Work out the finished part from the listing and answer in its coordinate system (mm). A direction names the side the tool comes from. Coordinates: 2 decimals unless noted, no trailing zeros. Write item = value, one per line. Start each with the question number.
Q1. Determine the mould class of faces 1 (the flat face through (17.5, -1, 48)), 2 (the cylindrical face through (0.245, 37.269, 35.107)), 3 (the cylindrical face through (0.245, 42.898, -55.946)) for opening direction Y: released by +Y, released by -Y, zero draft, split by the parting line, or undercut.
Q2. Find section A-A on x = -3. Give the number of separate pieces and of enclosed holes in the cut face, and give its area (3 significant figures).
Q3. Each of these flat-tipped pins is pushed along its axis until it touches: P1, Ø12, axis at x = -13.5, z = 45.5, coming from the -Y side; P2, Ø3, axis at x = -10, y = -50.5, coming from the +Z side; P3, Ø4, axis at x = 7.5, z = 46, coming from the +Y side. Where does it stop, or does it pass through?
Q4. Straight lines are drawn through the part: line 1 along Z through (x, y) = (15, -31); line 2 along Y through (x, z) = (8, -28); line 3 along Y through (x, z) = (-2, -62). For each, find the intervals that lie inside material, in ascending order.
Q5. A tool of negligible diameter and unlimited length cuts with its end or side. For faces 4 (the cylindrical face through (-11.239, 19.653, -45.292)), 5 (the cylindrical face through (11.2, 10.1, 55.6)), 6 (the cylindrical face through (0.245, 52.184, 26.527)), from which of +Z, -Z, +X, -X, +Y, -Y can it reach the whole face along a straight path? Write none if from no direction.
```python
from build123d import *

# Parameters (mm, degrees)
SKETCH1_W             = 35
SKETCH1_H             = 5
SKETCH7_R             = 46.2
REINFORCEMENT_DEPTH   = 35
SKETCH8_R             = 4
INSERTS_HOLES_A_DEPTH = 12.7


with BuildPart() as part:
    # Sketch1 → Body (revolve)
    with BuildSketch(Plane(origin=(0, 0, 0), x_dir=(1, 0, 0), z_dir=(0, 1, 0)), mode=Mode.PRIVATE) as body_sk:
        with Locations((0, 68)):
            Rectangle(SKETCH1_W, SKETCH1_H)
    revolve(body_sk.sketch.rotate(Axis((-1000, 0, 0), (1, 0, 0)), 180), axis=Axis((-1000, 0, 0), (1, 0, 0)))

    # Sketch7 → Reinforcement (add)
    with BuildSketch(Plane.ZY.offset(-17.5)):
        with BuildLine():
            ThreePointArc((15.227788826, 63.705293716), (7.666591863, 65.049776089), (0, 65.5))
            ThreePointArc((0, 65.5), (3.008755476, 58.35), (0, 51.2))
            ThreePointArc((0, 51.2), (-4.264821355, 51.022066783), (-8.5, 50.48950386))
            ThreePointArc((-8.5, 50.48950386), (-7.314547286, 58.179485578), (-12, 64.391381411))
            ThreePointArc((-12, 64.391381411), (-19.454347387, 62.544211305), (-26.641250121, 59.837227476))
            ThreePointArc((-26.641250121, 59.837227476), (-20.984448226, 54.529148555), (-20.824916125, 46.773527431))
            ThreePointArc((-20.824916125, 46.773527431), (-24.648652343, 44.876318228), (-28.3010677, 42.667195444))
            ThreePointArc((-28.3010677, 42.667195444), (-30.345900107, 50.17451037), (-37.15287981, 53.943614282))
            ThreePointArc((-37.15287981, 53.943614282), (-43.211453237, 49.22418419), (-48.675986069, 43.828054717))
            ThreePointArc((-48.675986069, 43.828054717), (-41.349250191, 41.279711944), (-38.049015064, 34.259487046))
            ThreePointArc((-38.049015064, 34.259487046), (-40.770507414, 30.971046563), (-43.208623688, 27.467341316))
            ThreePointArc((-43.208623688, 27.467341316), (-48.130171117, 33.493906497), (-55.881689177, 34.168506182))
            ThreePointArc((-55.881689177, 34.168506182), (-59.496906258, 27.392848441), (-62.294201817, 20.240613132))
            ThreePointArc((-62.294201817, 20.240613132), (-54.564391152, 20.892638123), (-48.694093634, 15.821670112))
            ThreePointArc((-48.694093634, 15.821670112), (-49.842771366, 11.710599583), (-50.645016102, 7.518134342))
            ThreePointArc((-50.645016102, 7.518134342), (-57.592298291, 11.021901908), (-64.948046817, 8.485352952))
            ThreePointArc((-64.948046817, 8.485352952), (-65.494803675, 0.82504034), (-65.141184147, -6.846614344))
            ThreePointArc((-65.141184147, -6.846614344), (-58.344853181, -3.106962633), (-50.919521043, -5.351857319))
            ThreePointArc((-50.919521043, -5.351857319), (-50.29676734, -9.574716451), (-49.324425137, -13.73102636))
            ThreePointArc((-49.324425137, -13.73102636), (-57.096193882, -13.355889651), (-62.784297127, -18.664994891))
            ThreePointArc((-62.784297127, -18.664994891), (-60.168054535, -25.88542473), (-56.724663948, -32.75))
            ThreePointArc((-56.724663948, -32.75), (-52.036960049, -26.569341324), (-44.340500674, -25.6))
            ThreePointArc((-44.340500674, -25.6), (-42.05399531, -29.204477028), (-39.475192967, -32.605967862))
            ThreePointArc((-39.475192967, -32.605967862), (-46.727638847, -35.424326556), (-49.764572087, -42.587995551))
            ThreePointArc((-49.764572087, -42.587995551), (-44.437702156, -48.120064704), (-38.499934025, -52.990613132))
            ThreePointArc((-38.499934025, -52.990613132), (-36.731403783, -45.437639525), (-30.094604917, -41.421670112))
            ThreePointArc((-30.094604917, -41.421670112), (-26.539705442, -43.784518212), (-22.800341312, -45.843041305))
            ThreePointArc((-22.800341312, -45.843041305), (-28.279450549, -51.367575579), (-28.140100436, -59.14714488))
            ThreePointArc((-28.140100436, -59.14714488), (-21.023667371, -62.034308332), (-13.618215749, -64.068667848))
            ThreePointArc((-13.618215749, -64.068667848), (-15.074654109, -56.449357065), (-10.64507857, -50.081157158))
            ThreePointArc((-10.64507857, -50.081157158), (-6.436459398, -50.793818427), (-2.18310351, -51.153436435))
            ThreePointArc((-2.18310351, -51.153436435), (-4.94148834, -58.428904124), (-1.649949774, -65.479215525))
            ThreePointArc((-1.649949774, -65.479215525), (6.025550497, -65.222256487), (13.618215749, -64.068667848))
            ThreePointArc((13.618215749, -64.068667848), (9.18864021, -57.700467941), (10.64507857, -50.081157158))
            ThreePointArc((10.64507857, -50.081157158), (14.77970895, -49.020405989), (18.811612722, -47.618937691))
            ThreePointArc((18.811612722, -47.618937691), (19.250902095, -55.387344337), (25.125492192, -60.489334945))
            ThreePointArc((25.125492192, -60.489334945), (32.032895944, -57.132683969), (38.499934025, -52.990613132))
            ThreePointArc((38.499934025, -52.990613132), (31.86313516, -48.974643718), (30.094604917, -41.421670112))
            ThreePointArc((30.094604917, -41.421670112), (33.440331351, -38.770920019), (36.553630216, -35.850692016))
            ThreePointArc((36.553630216, -35.850692016), (40.114636669, -42.768809535), (47.556508301, -45.040298825))
            ThreePointArc((47.556508301, -45.040298825), (52.501462672, -39.164351358), (56.724663948, -32.75))
            ThreePointArc((56.724663948, -32.75), (49.028204573, -31.780658676), (44.340500674, -25.6))
            ThreePointArc((44.340500674, -25.6), (46.318816665, -21.817589755), (47.975192967, -17.883535998))
            ThreePointArc((47.975192967, -17.883535998), (54.042186133, -22.755159023), (61.764572087, -21.80338586))
            ThreePointArc((61.764572087, -21.80338586), (63.892049543, -14.424146601), (65.141184147, -6.846614344))
            ThreePointArc((65.141184147, -6.846614344), (57.715852009, -9.09150903), (50.919521043, -5.351857319))
            ThreePointArc((50.919521043, -5.351857319), (51.188357785, -1.091800016), (51.101409013, 3.175845861))
            ThreePointArc((51.101409013, 3.175845861), (58.625350656, 1.193065209), (65.292980245, 5.203530598))
            ThreePointArc((65.292980245, 5.203530598), (64.235120607, 12.810124142), (62.294201817, 20.240613132))
            ThreePointArc((62.294201817, 20.240613132), (56.4239043, 15.169645121), (48.694093634, 15.821670112))
            ThreePointArc((48.694093634, 15.821670112), (47.206966812, 19.822771865), (45.391727198, 23.686095119))
            ThreePointArc((45.391727198, 23.686095119), (53.071659457, 24.934997627), (57.531638952, 31.310709343))
            ThreePointArc((57.531638952, 31.310709343), (53.471355761, 37.829408046), (48.675986069, 43.828054717))
            ThreePointArc((48.675986069, 43.828054717), (45.375750942, 36.807829818), (38.049015064, 34.259487046))
            ThreePointArc((38.049015064, 34.259487046), (35.063062416, 37.309806406), (31.83340338, 40.100803349))
            ThreePointArc((31.83340338, 40.100803349), (38.341396196, 44.365442429), (39.822554625, 52.003981993))
            ThreePointArc((39.822554625, 52.003981993), (33.461907731, 56.307643628), (26.641250121, 59.837227476))
            ThreePointArc((26.641250121, 59.837227476), (26.481718021, 52.081606351), (20.824916125, 46.773527431))
            ThreePointArc((20.824916125, 46.773527431), (16.856435989, 48.34563647), (12.770794921, 49.581718376))
            ThreePointArc((12.770794921, 49.581718376), (16.981557213, 56.124699187), (15.227788826, 63.705293716))
        make_face()
        with Locations(Location((0, 0, 0), (0, 0, 180))):
            Circle(SKETCH7_R, mode=Mode.SUBTRACT)
    extrude(amount=REINFORCEMENT_DEPTH)

    # Sketch8 → Inserts_Holes_A (cut)
    with BuildSketch(Plane.ZY.offset(17.5)):
        with Locations((7.5, 52)):
            Circle(SKETCH8_R)
        with Locations((51.772566305, 8.935959835)):
            Circle(SKETCH8_R)
        with Locations((24.497205661, -46.4772731)):
            Circle(SKETCH8_R)
        with Locations((-36.632460577, -37.660494315)):
            Circle(SKETCH8_R)
        with Locations((-47.13731139, 23.20180758)):
            Circle(SKETCH8_R)
    inserts_holes_a = extrude(amount=-INSERTS_HOLES_A_DEPTH, mode=Mode.SUBTRACT)

    # Mirror1: Inserts_Holes_A across plane
    add(inserts_holes_a.mirror(Plane(origin=(0, 0, 0), x_dir=(0, 0, 1), z_dir=(1, 0, 0))), mode=Mode.SUBTRACT)


solid = part.part
```
Findings below:
q1.face_1 = zero draft
q1.face_2 = undercut
q1.face_3 = split by the parting line
q2.separate_pieces = 1
q2.enclosed_holes = 16
q2.area = 6,700 mm^2
q3.P1 = -58.4
q3.P2 = 50.69
q3.P3 = 55.08
q4.line_1 = -63.32 to -56.1, -40.75 to -34.26, 34.26 to 47.87, 57.7 to 63.32
q4.line_2 = -64.7 to -50.74, -42.87 to -36.75, 36.75 to 42.87, 59.21 to 64.7
q4.line_3 = -33.56 to -17.24, -4.23 to 10.32, 20.39 to 33.56
q5.face_4 = -X
q5.face_5 = +X
q5.face_6 = +X, -X
